Could you check a few things on this drawing? It's one solid part, dimensions in mm from its lowest x, y, z. A direction names the side the tool comes from. Give positions to 0.01 mm unless a question says otherwise; leave off trailing zeros. Loops run counter-clockwise (first coordinate to the right, second up) from the corner with the lowest first, then second, coordinate; pieces in that order, holes last. Notation, with made-up numbers: (33.25, 70) - (43.25, 70) arc R28 ccw to (43.25, 106) - close; hole circle Ø1 at (51, 46). An arc over 180 degrees is marked (long way). Answer as a JSON object with one key per item and string values.
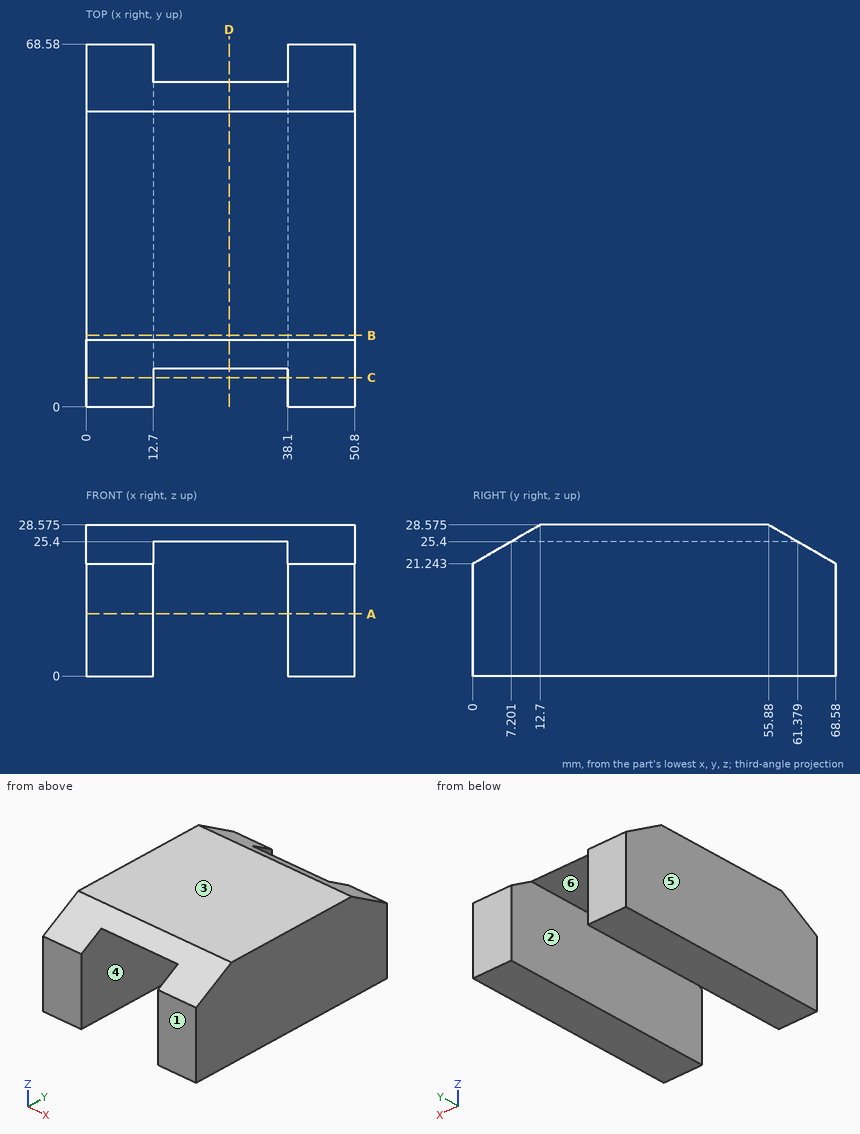
1) Imagine slicing it at C-C on y = 5.5. Write out the boundary of the cut face in (x, z).
Check sheet entries:
{"outline": "(0, 0) - (12.7, 0) - (12.7, 24.42) - (0, 24.42) - close; (38.1, 0) - (50.8, 0) - (50.8, 24.42) - (38.1, 24.42) - close"}
2) I'm going to push a flat-ended pin straight in: P1, Ø7.5, axis at x = 20, y = 47, coming from the -Z side. Where does the tip first touch, or does it pass through?
Check sheet entries:
{"P1": "z = 25.4"}
3) Imagine slicing it at A-A on z = 11.75. Write out the boundary of the cut face in (x, y).
Check sheet entries:
{"outline": "(0, 0) - (12.7, 0) - (12.7, 68.58) - (0, 68.58) - close; (38.1, 0) - (50.8, 0) - (50.8, 68.58) - (38.1, 68.58) - close"}
4) Imagine slicing it at B-B on y = 13.5. Write out the boundary of the cut face in (x, z) (1 decimal).
Check sheet entries:
{"outline": "(0, 0) - (12.7, 0) - (12.7, 25.4) - (38.1, 25.4) - (38.1, 0) - (50.8, 0) - (50.8, 28.6) - (0, 28.6) - close"}
5) I need wall thicknesses on L1, parallel to X at y = 38.5, z = 10.25; L2, parallel to Z at x = 28.5, y = 20.5 (1 decimal); L3, parallel to Z at x = 7, y = 62. Which ranges of each line are inside material? Lowest first, please.
Check sheet entries:
{"L1": "0 to 12.7, 38.1 to 50.8", "L2": "25.4 to 28.6", "L3": "0 to 25.04"}
6) If we mould it in two halves opening along X, with no side actions, what happens to the marked faces 3, 4, 5 and 6? For each: released by +X, released by -X, zero draft, split by the parting line, or undercut.
Check sheet entries:
{"face 3": "zero draft", "face 4": "undercut", "face 5": "released by -X", "face 6": "undercut"}
7) Imagine slicing it at D-D on x = 27. Write out the boundary of the cut face in (y, z) (1 decimal).
Check sheet entries:
{"outline": "(7.2, 25.4) - (61.4, 25.4) - (55.9, 28.6) - (12.7, 28.6) - close"}
8) Which directions (+Z, -Z, +X, -X, +Y, -Y) give clear straight access to the entire face, cutting with the end or side of a thin tool? Please do the marked faces 1 and 2.
Check sheet entries:
{"face 1": "+Z, -Z, +X, -X, -Y", "face 2": "-Z, +Y, -Y"}
